Build history of the part. All positions in model axes, mm. A direction names the side the tool comes from. Give positions to 0.01 mm unless a question says otherwise; leave off trailing zeros. Order: outer loops, then holes, each group sorted by start corner. A loop starts at its lowest first (then second) coordinate and runs counter-clockwise, first axis right, second up. Notation, with made-up numbers: (32, 59.25) -> (37, 59.25) arc R13 ccw to (37, 75.25) -> close; hole circle Ø4 at (25, 85.25). An arc over 180 degrees is marked (long way). One line per item, written item: value. Start each with the question number.
(1) Saw through at D-D on z = 36. Give the cut face in (x, y).
(2) Two-plate mould, pull along Y, no slides. Class faces 4 (the flat face through (-10, 50, 10)), 5 (the cylindrical face through (-89.86, 26.299, 56.185)), 6 (the cylindrical face through (-0.57, 2.46, 0.6)): +Y half, -Y half, draft (parallel to the pull), parting line (faces both ways), or undercut.
(3) Saw through at C-C on y = 40.5. Give the cut face in (x, z).
(4) Saw through at B-B on x = -50. Give the cut face in (y, z).
(5) Pin check, flat tip, straight feed: pin 1 (8 mm diameter, centred on x = -56, z = 7, fed in from +Y). Stop position of the tip, or through.
(6) Which spindle directions (+Z, -Z, +X, -X, +Y, -Y) get a long thin tool onto all of the face, cutting with end or side? Do faces 1 (the cylindrical face through (-39.862, 2.465, 24.944)), 2 (the flat face through (-10, 27, 20)), 3 (the flat face through (-80, 27.8, 64.3)). Say none if no direction does.
(7) Saw through at A-A on z = 45. Give the cut face in (x, y).
(8) Probe line 1 (X direction, y = 1.95, z = 36); line 2 (Y direction, x = -92, z = 10); line 3 (Z direction, x = -84.5, y = 34.5). List the from-to ranges inside material, lowest first.
```python
from build123d import *

# Parameters (mm, degrees)
SKETCH1_R           = 15
SKETCH1_R_2         = 4
BOSS_EXTRUDE1_DEPTH = 5
SKETCH4_W           = 20
SKETCH4_H           = 45
SKETCH4_R           = 4
BOSS_EXTRUDE2_DEPTH = 20
BOSS_EXTRUDE3_START = -20
SKETCH6_W           = 20
SKETCH6_H           = 45
SKETCH6_R           = 4
BOSS_EXTRUDE3_DEPTH = 20
FILLET1_R           = 2
FILLET2_R           = 2
FILLET3_R           = 2


with BuildPart() as part:
    # Sketch1 → Boss-Extrude1 (new body)
    with BuildSketch(Plane(origin=(0, 0, 0), x_dir=(1, 0, 0), z_dir=(0, 1, 0))):
        with BuildLine():
            Line((-2, 0), (-98, 0))
            ThreePointArc((-98, 0), (-99.414213562, -0.585786438), (-100, -2))
            Line((-100, -2), (-100, -68))
            ThreePointArc((-100, -68), (-99.414213562, -69.414213562), (-98, -70))
            Line((-98, -70), (-2, -70))
            ThreePointArc((-2, -70), (-0.585786438, -69.414213562), (0, -68))
            Line((0, -68), (0, -2))
            ThreePointArc((0, -2), (-0.585786438, -0.585786438), (-2, 0))
        make_face()
        with Locations(Location((-50, -36, 0), (0, 0, 270))):
            Circle(SKETCH1_R, mode=Mode.SUBTRACT)
        with Locations(Location((-35, -21, 0), (0, 0, 270))):
            Circle(SKETCH1_R_2, mode=Mode.SUBTRACT)
        with Locations(Location((-65, -21, 0), (0, 0, 270))):
            Circle(SKETCH1_R_2, mode=Mode.SUBTRACT)
        with Locations(Location((-65, -50.396825397, 0), (0, 0, 270))):
            Circle(SKETCH1_R_2, mode=Mode.SUBTRACT)
        with Locations(Location((-35, -51, 0), (0, 0, 270))):
            Circle(SKETCH1_R_2, mode=Mode.SUBTRACT)
        with Locations(Location((-50, -14.786796564, 0), (0, 0, 270))):
            Circle(SKETCH1_R_2, mode=Mode.SUBTRACT)
        with Locations(Location((-28.786796564, -36, 0), (0, 0, 270))):
            Circle(SKETCH1_R_2, mode=Mode.SUBTRACT)
        with Locations(Location((-50, -57.213203436, 0), (0, 0, 270))):
            Circle(SKETCH1_R_2, mode=Mode.SUBTRACT)
        with Locations(Location((-71.213203436, -36, 0), (0, 0, 270))):
            Circle(SKETCH1_R_2, mode=Mode.SUBTRACT)
    extrude(amount=BOSS_EXTRUDE1_DEPTH)

    # Sketch4 → Boss-Extrude2 (add)
    # profile 1 of 2: a face of its own
    with BuildSketch(Plane(origin=(0, 0, 0), x_dir=(0, 0, -1), z_dir=(1, 0, 0))):
        with Locations((-10, 27.5)):
            Rectangle(SKETCH4_W, SKETCH4_H)
        with Locations((-10, 27.5)):
            Circle(SKETCH4_R, mode=Mode.SUBTRACT)
    # profile 2 of 2: a face of its own
    with BuildSketch(Plane(origin=(0, 0, 0), x_dir=(0, 0, -1), z_dir=(1, 0, 0))):
        with Locations((-60, 27.5)):
            Rectangle(SKETCH4_W, SKETCH4_H)
        with Locations((-60, 27.5)):
            Circle(SKETCH4_R, mode=Mode.SUBTRACT)
    extrude(amount=-BOSS_EXTRUDE2_DEPTH)

    # Sketch6 → Boss-Extrude3 (add)
    # profile 1 of 2: a face of its own
    with BuildSketch(Plane.ZY.offset(100).offset(BOSS_EXTRUDE3_START)):
        with Locations((10, 27.5)):
            Rectangle(SKETCH6_W, SKETCH6_H)
        with Locations(Location((10, 27.5, 0), (0, 0, 180))):
            Circle(SKETCH6_R, mode=Mode.SUBTRACT)
    # profile 2 of 2: a face of its own
    with BuildSketch(Plane.ZY.offset(100).offset(BOSS_EXTRUDE3_START)):
        with Locations((60, 27.5)):
            Rectangle(SKETCH6_W, SKETCH6_H)
        with Locations(Location((60, 27.5, 0), (0, 0, 180))):
            Circle(SKETCH6_R, mode=Mode.SUBTRACT)
    extrude(amount=BOSS_EXTRUDE3_DEPTH)

    # Fillet1
    fillet1_edges = [part.edges().sort_by_distance(p)[0] for p in [
        (-100, 27.5, 70),
        (-100, 27.5, 0),
    ]]
    fillet(fillet1_edges, radius=FILLET1_R)

    # Fillet2
    fillet2_edges = [part.edges().sort_by_distance(p)[0] for p in [
        (0, 27.5, 0),
    ]]
    fillet(fillet2_edges, radius=FILLET2_R)

    # Fillet3
    fillet3_edges = [part.edges().sort_by_distance(p)[0] for p in [
        (0, 27.5, 70),
    ]]
    fillet(fillet3_edges, radius=FILLET3_R)


solid = part.part
```
Results below:
1. outline: (-100, 0) -> (-75.21, 0) -> (-75.21, 5) -> (-100, 5) -> close; (-67.21, 0) -> (-65, 0) -> (-65, 5) -> (-67.21, 5) -> close; (-35, 0) -> (-32.79, 0) -> (-32.79, 5) -> (-35, 5) -> close; (-24.79, 0) -> (0, 0) -> (0, 5) -> (-24.79, 5) -> close
2. face 4: +Y half
2. face 5: undercut
2. face 6: draft
3. outline: (-100, 2) arc R2 ccw to (-98, 0) -> (-80, 0) -> (-80, 20) -> (-100, 20) -> close; (-100, 50) -> (-80, 50) -> (-80, 70) -> (-98, 70) arc R2 ccw to (-100, 68) -> close; (-20, 0) -> (-2, 0) arc R2 ccw to (0, 2) -> (0, 20) -> (-20, 20) -> close; (-20, 50) -> (0, 50) -> (0, 68) arc R2 ccw to (-2, 70) -> (-20, 70) -> close
4. outline: (0, 0) -> (5, 0) -> (5, 10.79) -> (0, 10.79) -> close; (0, 18.79) -> (5, 18.79) -> (5, 21) -> (0, 21) -> close; (0, 51) -> (5, 51) -> (5, 53.21) -> (0, 53.21) -> close; (0, 61.21) -> (5, 61.21) -> (5, 70) -> (0, 70) -> close
5. pin 1: stops at y = 5
6. face 1: +Y, -Y
6. face 2: +X, -X, +Y
6. face 3: +Z, -Z, +Y
7. outline: (-100, 0) -> (-62, 0) -> (-62, 5) -> (-100, 5) -> close; (-38, 0) -> (0, 0) -> (0, 5) -> (-38, 5) -> close
8. line 1: x = -100 to -75.21, -67.21 to -65, -35 to -32.79, -24.79 to 0
8. line 2: y = 0 to 23.5, 31.5 to 50
8. line 3: z = 0 to 20, 50 to 70
